Autodesk Fusion 360 part; units mm, degrees
sketch "Sketch1" plane through (0, 0, 0) normal (0, 0, 1) x (1, 0, 0)
  line L0 (0, 0) -> (60, 0)
  line L1 (60, 0) -> (60, -60)
  line L2 (60, -60) -> (0, -60)
  line L3 (0, -60) -> (0, 0)
  dimension "d1" = 60
  dimension "d2" = 60
extrude "Extrude1" add sketch "Sketch1" along normal blind 2
sketch "Sketch2" plane through (0, 0, 2) normal (0, 0, 1) x (-1, 0, 0)
  line L0 (0, 60) -> (-60, 60)
  line L1 (-60, 60) -> (-60, 0)
  line L2 (-60, 0) -> (0, 0)
  line L3 (0, 0) -> (0, 60)
  line L4 (-60, 10) -> (-56.5, 10)
  line L5 (-60, 3.5) -> (-50, 3.5)
  line L6 (-30, 0) -> (-30, 60)
  line L7 (0, 30) -> (-60, 30)
  line L8 (-30, 0) -> (-30, 3.5)
  line L9 (0, 30) -> (-3.5, 30)
  line L10 (-60, 30) -> (-56.5, 30)
  point P0 (-10, 3.5)
  point P1 (-3.5, 10)
  point P2 (-3.5, 50)
  point P3 (-10, 56.5)
  point P4 (-50, 56.5)
  point P5 (-56.5, 50)
  point P6 (-30, 56.5)
  dimension "d5" = 3.5
  dimension "d6" = 10
  dimension "d7" = 10
  dimension "d8" = 3.5
  dimension "d9" = 3.5
  dimension "d10" = 3.5
  dimension "d11" = 3.5
hole "Hole1" at (10, -3.5, 2) at (3.5, -10, 2) at (3.5, -30, 2) at (3.5, -50, 2) at (10, -56.5, 2) at (30, -56.5, 2) at (50, -56.5, 2) at (56.5, -50, 2) at (56.5, -30, 2) at (56.5, -10, 2) at (50, -3.5, 2) at (30, -3.5, 2) direction (0, 0, -1) diameter 4 depth 50 tip angle 180
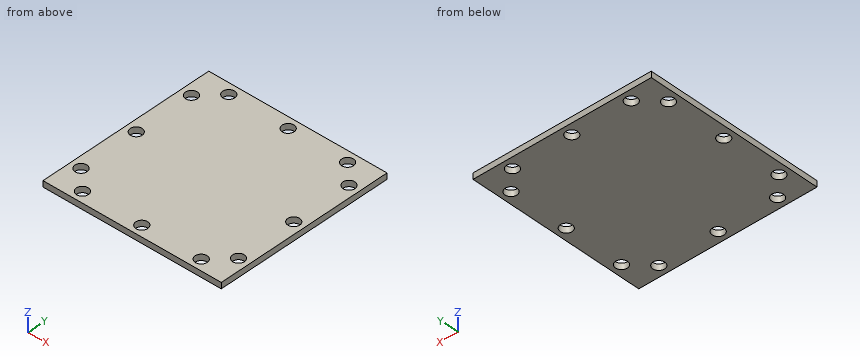
The model under review builds one solid part; all positions refer to its coordinate system, in mm. Round coordinates to 2 decimals unless told otherwise and drop trailing zeros. Loops run counter-clockwise (first coordinate to the right, second up) from the corner with the lowest first, then second, coordinate; pieces in that order, holes last. Notation, with made-up numbers: (41.25, 75) -> (48.25, 75) arc R8 cw to (48.25, 83) -> close; hole circle Ø9 at (-21.75, -2). An arc over 180 degrees is marked (long way). Write item = value, one per line. Start each with the question number.
Item 1: Take a section at C-C on x = 3.5. Give the boundary of the cut face in (y, z).
Item 2: To check wall thickness, follow L1, parallel to Y at x = 56.5, z = 1.15; L2, parallel to X at y = -3.5, z = 1.15; L3, parallel to X at y = -50, z = 0.5. State the ranges of each line that lie inside material, in increasing order.
Item 3: Take a section at A-A on z = 0.6. Count the separate pieces of the cut face and the enclosed holes in it, plus the area to 3 significant figures.
Item 4: Take a section at D-D on x = 30. Give the boundary of the cut face in (y, z), plus the area to 3 significant figures.
Item 5: Take a section at B-B on y = -56.5. Give the boundary of the cut face in (x, z).
Result:
q1.outline = (-60, 0) -> (-52, 0) -> (-52, 2) -> (-60, 2) -> close; (-48, 0) -> (-32, 0) -> (-32, 2) -> (-48, 2) -> close; (-28, 0) -> (-12, 0) -> (-12, 2) -> (-28, 2) -> close; (-8, 0) -> (0, 0) -> (0, 2) -> (-8, 2) -> close
q2.L1 = -60 to -52, -48 to -32, -28 to -12, -8 to 0
q2.L2 = 0 to 8, 12 to 28, 32 to 48, 52 to 60
q2.L3 = 0 to 1.5, 5.5 to 54.5, 58.5 to 60
q3.separate_pieces = 1
q3.enclosed_holes = 12
q3.area = 3,450 mm²
q4.outline = (-60, 0) -> (-58.5, 0) -> (-58.5, 2) -> (-60, 2) -> close; (-54.5, 0) -> (-5.5, 0) -> (-5.5, 2) -> (-54.5, 2) -> close; (-1.5, 0) -> (0, 0) -> (0, 2) -> (-1.5, 2) -> close
q4.area = 104 mm²
q5.outline = (0, 0) -> (8, 0) -> (8, 2) -> (0, 2) -> close; (12, 0) -> (28, 0) -> (28, 2) -> (12, 2) -> close; (32, 0) -> (48, 0) -> (48, 2) -> (32, 2) -> close; (52, 0) -> (60, 0) -> (60, 2) -> (52, 2) -> close
